Verification items for the finished model (mm, model axes). Face numbers are marked on the shaded views. A direction names the side the tool comes from. Give positions to 0.01 mm unless a question says otherwise; leave off trailing zeros. Write each loop counter-clockwise with the first axis right and the second up, starting at its lowest first coordinate (ties: lowest second). Pieces come first, ordered by that corner, then holes. Notation, with made-up numbers: (9, 33.5) -> (42, 33.5) arc R14 cw to (42, 50.5) -> close; hole circle Ø2 at (11.25, -2.75). An arc over 180 degrees is marked (long way). Use one line per item in the form item = value. Start each with the question number.
(1) Set-up check for the marked faces 1, 2 and 3: record each of +Z, -Z, +X, -X, +Y, -Y from which the full face is reachable in a straight line by a thin tool's end or side.
(2) Section check C-C, the plane z = 37.5. Record the cut outline in (x, y), plus the area to 3 significant figures.
(3) Scan lines: L1, parallel to Z at x = 0, y = 55.5; L2, parallel to X at y = 59, z = 40; L3, parallel to X at y = 73, z = 25. Record each from-to range of solid material in increasing order.
(4) Depth check by flat-ended pin: pin 1 Ø22.5 at (x, y) = (72, 57) entering from +Z; pin 2 Ø11.5 at (y, z) = (43.5, 16) entering from -X; pin 3 Ø6 at (x, z) = (-61.5, 4.5) entering from +Y; pin 4 Ø11.5 at (y, z) = (19.5, 14) entering from +X. Enter the tip coordinate at first touch or a pass-through.
(5) Section check A-A, the plane y = 30.5. Record the cut outline in (x, z).
(6) Section check D-D, the plane x = 68. Record the cut outline in (y, z).
(7) Section check B-B, the plane x = 0. Record the cut outline in (y, z), plus the area to 3 significant figures.
(8) Release check for a two-part mould opening along X. For the marked faces 4, 5, 6 and 7 record: pulls with the +X half, pulls with the -X half, needs draft (parallel to the pull), parting line crosses it, or undercut.
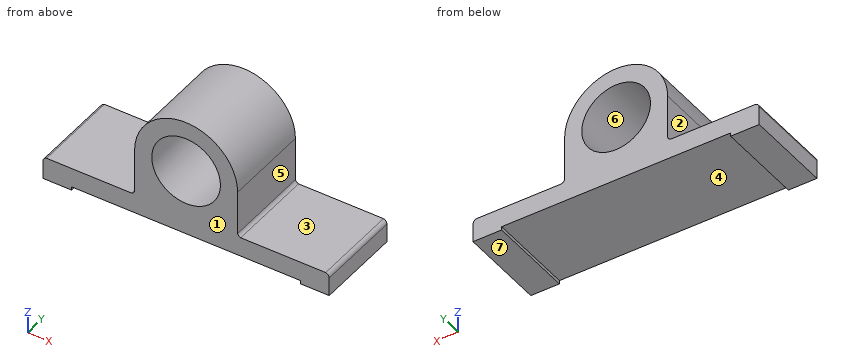
from build123d import *

# Parameters (mm, degrees)
F0_R     = 30
F1_DEPTH = 76.2


with BuildPart() as f1:
    # F0 (on Front) → F1 (new body)
    with BuildSketch(Plane.XZ):
        with BuildLine():
            Line((45, 2.903346), (45, 41.171368))
            ThreePointArc((45, 41.171368), (0, 86.171368), (-45, 41.171368))
            Line((-45, 41.171368), (-45, 2.903346))
            ThreePointArc((-45, 2.903346), (-46.008278, 1.202846), (-47.707793, 0.192909))
            Line((-47.707793, 0.192909), (-121.913321, 0.192909))
            ThreePointArc((-121.913321, 0.192909), (-124.058806, -1.116044), (-125, -3.446413))
            Line((-125, -3.446413), (-125, -19.807091))
            Line((-125, -19.807091), (-100, -19.807091))
            Line((-100, -19.807091), (-100, -16.807091))
            Line((-100, -16.807091), (0, -16.807091))
            Line((0, -16.807091), (100, -16.807091))
            Line((100, -16.807091), (100, -19.807091))
            Line((100, -19.807091), (125, -19.807091))
            Line((125, -19.807091), (125, -3.446413))
            ThreePointArc((125, -3.446413), (124.058806, -1.116044), (121.913321, 0.192909))
            Line((121.913321, 0.192909), (47.707793, 0.192909))
            ThreePointArc((47.707793, 0.192909), (46.008278, 1.202846), (45, 2.903346))
        make_face()
        with Locations((0, 41.171368)):
            Circle(F0_R, mode=Mode.SUBTRACT)
    extrude(amount=-F1_DEPTH)


solid = f1.part
Completed:
q1.face_1 = +Z, -Z, +X, -X, -Y
q1.face_2 = +Z, -X, +Y, -Y
q1.face_3 = +Z, +X, +Y, -Y
q2.outline = (-45, 0) -> (-29.77, 0) -> (-29.77, 76.2) -> (-45, 76.2) -> close; (29.77, 0) -> (45, 0) -> (45, 76.2) -> (29.77, 76.2) -> close
q2.area = 2,320 mm²
q3.L1 = -16.81 to 11.17, 71.17 to 86.17
q3.L2 = -45 to -29.98, 29.98 to 45
q3.L3 = -45 to -25.27, 25.27 to 45
q4.pin_1 = 0.19
q4.pin_2 = -45
q4.pin_3 = through
q4.pin_4 = 45
q5.outline = (-125, -19.81) -> (-100, -19.81) -> (-100, -16.81) -> (100, -16.81) -> (100, -19.81) -> (125, -19.81) -> (125, -3.45) arc R4 ccw to (121.91, 0.19) -> (47.71, 0.19) arc R4 cw to (45, 2.9) -> (45, 41.17) arc R45 ccw to (-45, 41.17) -> (-45, 2.9) arc R4 cw to (-47.71, 0.19) -> (-121.91, 0.19) arc R4 ccw to (-125, -3.45) -> close; hole circle Ø60 at (0, 41.17)
q6.outline = (0, -16.81) -> (76.2, -16.81) -> (76.2, 0.19) -> (0, 0.19) -> close
q7.outline = (0, -16.81) -> (76.2, -16.81) -> (76.2, 11.17) -> (0, 11.17) -> close; (0, 71.17) -> (76.2, 71.17) -> (76.2, 86.17) -> (0, 86.17) -> close
q7.area = 3,270 mm²
q8.face_4 = undercut
q8.face_5 = pulls with the +X half
q8.face_6 = undercut
q8.face_7 = needs draft
